```python
from build123d import *

# Parameters (mm, degrees)
SKETCH_1_R          = 10
EXTRUDE_1_DEPTH     = 25
SKETCH_2_R          = 3.3
CUT_EXTRUDE_1_DEPTH = 12
FILLET_1_R          = 1
SKETCH_3_R          = 2
CUT_EXTRUDE_2_DEPTH = 29.722813268


with BuildPart() as part:
    # 草图1 → 凸台-拉伸1 (new body)
    with BuildSketch(Plane.XY):
        Circle(SKETCH_1_R)
    extrude(amount=EXTRUDE_1_DEPTH)

    # 草图2 → 切除-拉伸1 (cut)
    with BuildSketch(Plane.XY.offset(25)):
        Circle(SKETCH_2_R)
    extrude(amount=-CUT_EXTRUDE_1_DEPTH, mode=Mode.SUBTRACT)

    # 圆角1
    fillet_1_edges = [part.edges().sort_by_distance(p)[0] for p in [
        (-10, 0, 0),
        (-10, 0, 25),
    ]]
    fillet(fillet_1_edges, radius=FILLET_1_R)

    # 草图3 → 切除-拉伸2 (cut, through all)
    with BuildSketch(Plane(origin=(0, 0, 0), x_dir=(-1, 0, 0), z_dir=(0, 0, -1))):
        Circle(SKETCH_3_R)
    extrude(amount=-CUT_EXTRUDE_2_DEPTH, mode=Mode.SUBTRACT)


solid = part.part
```
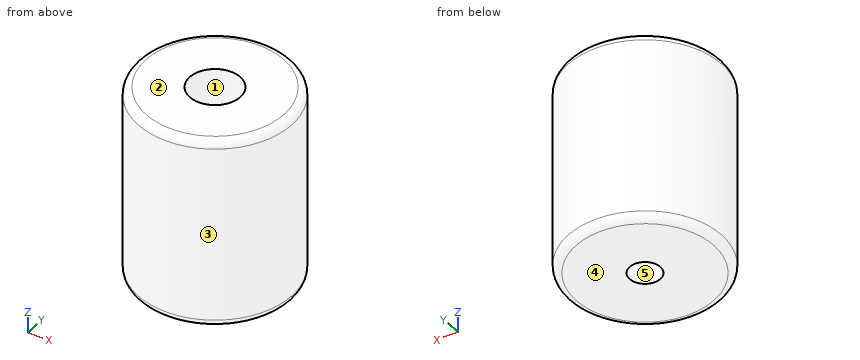
The listing builds one solid part. Answer for the finished solid, in the listing's coordinates (mm). Face numbers are marked on the shaded views. A direction names the side the tool comes from. Coordinates: 2 decimals unless noted, no trailing zeros. Order: outer loops, then holes, each group sorted by start corner. A loop starts at its lowest first (then second) coordinate and runs counter-clockwise, first axis right, second up. Notation, with made-up numbers: M -5.5,57 L 18.5,57 A14 cw 18.5,81 Z; hole C -2.5,73.5 d11. An arc over 180 degrees is marked long. Answer as a JSON object with one key per item and string values. Group by question number.
1. Section D-D on z = 13.5 is taken. Write down the section's boundary in (x, y), then the cut area to 3 significant figures.
2. Section C-C on z = 5 is taken. Write down the section's boundary in (x, y), then the cut area to 3 significant figures.
3. A tool of negligible diameter and unlimited length cuts with its end or side. For the marked faces 1 and 2, from which of +Z, -Z, +X, -X, +Y, -Y can it reach the whole face along a straight path? Write none if from no direction.
4. Straight lines are drawn through the part: line 1 (Y direction, x = 0, z = 22); line 2 (Y direction, x = 0, z = 6.75); line 3 (Z direction, x = 2.75, y = 1.75). For each, find the intervals that lie inside material, in ascending order.
5. Determine the mould class of the marked faces 3, 4 and 5 for opening direction X: released by +X, released by -X, zero draft, split by the parting line, or undercut.
6. Flat-ended cylindrical pins translate along their axes: P1, Ø3, axis at x = -3.5, z = 19.5, coming from the -Y side; P2, Ø1, axis at y = -2.5, z = 13, coming from the +X side; P3, Ø2.5, axis at x = 0, y = 0, coming from the -Z side; P4, Ø1, axis at y = 3, z = 7.5, coming from the +X side. Find the tip coordinate at first contact, or state that the pin passes through.
7. Section A-A on x = 0 is taken. Write down the section's boundary in (y, z).
Values follow:
{
 "1": {"outline": "C 0,0 d20; hole C 0,0 d6.6", "area": "280 mm2"},
 "2": {"outline": "C 0,0 d20; hole C 0,0 d4", "area": "302 mm2"},
 "3": {"face 1": "+Z", "face 2": "+Z, +X, -X, +Y, -Y"},
 "4": {"line 1": "-10 to -3.3, 3.3 to 10", "line 2": "-10 to -2, 2 to 10", "line 3": "0 to 13"},
 "5": {"face 3": "split by the parting line", "face 4": "zero draft", "face 5": "undercut"},
 "6": {"P1": "y = -9.8", "P2": "x = 9.8", "P3": "through", "P4": "x = 9.68"},
 "7": {"outline": "M -10,1 A1 ccw -9,0 L -2,0 L -2,13 L -3.3,13 L -3.3,25 L -9,25 A1 ccw -10,24 Z; M 2,0 L 9,0 A1 ccw 10,1 L 10,24 A1 ccw 9,25 L 3.3,25 L 3.3,13 L 2,13 Z"}
}
